Source: CAD feature listing. Evaluate the final solid. Frame: model axes, mm. A direction names the side the tool comes from. Coordinates: 2 decimals unless noted, no trailing zeros. Loops run counter-clockwise (first coordinate to the right, second up) from the corner with the lowest first, then second, coordinate; pieces in that order, holes last. Notation, with made-up numbers: M -36,7.25 L 23,7.25 A20 ccw 23,14.25 Z; hole C -8.75,23.25 d4. An arc over 180 degrees is marked long. One line per question, with ' | ' between items. Start each with the question number.
1. Section query B-B, the plane y = 4.5. Output: boundary loops of the cut face in (x, z).
2. Ray query, probe 1 along X at (y, z) = (3, 6); probe 2 along X at (y, z) = (-5.25, 6); probe 3 along X at (y, z) = (6.5, 6). Return the intervals inside material, ascending.
3. Section query A-A, the plane z = 6. Output: boundary loops of the cut face in (x, y).
4. Access query for faces 5 (the flat face through (9, 0, 1)), 6 (the flat face through (22, 10, 5)). Directions: +Z, -Z, +X, -X, +Y, -Y. A direction counts if a zero-diameter tool reaches every point of the face in a straight line with its end or side. Return the directions, or none.
5. Pin query (flat end, axial travel): P1, Ø4, axis at x = 5, z = 6.5, coming from the +Y side; P2, Ø6.5, axis at x = 12, z = 6, coming from the +Y side; P3, Ø5, axis at x = 17, z = 1.5, coming from the -Y side; P4, Ø1.5, axis at x = 13, y = -2, coming from the -Z side. Return the tip coordinate at first contact, or that it passes through.
6. Section query C-C, the plane x = 4. Output: boundary loops of the cut face in (y, z), and give its area (3 significant figures).
7. Mould query, pull axis Z, two halves, no side actions, for faces 1 (the flat face through (12, 4, 12)), 2 (the flat face through (12, 4, 0)), 3 (the flat face through (14, -10, 8)), 4 (the cylindrical face through (2.8, 5.1, 4.4)). Classes: pulls with the +Z half, pulls with the -Z half, needs draft (parallel to the pull), parting line crosses it, or undercut.
```python
from build123d import *

# Parameters (mm, degrees)
BOSS_EXTRUDE1_DEPTH = 12
SKETCH2_R           = 2
CUT_EXTRUDE1_DEPTH  = 29.635642127
SKETCH3_R           = 4.5
SKETCH3_R_2         = 2.5
BOSS_EXTRUDE2_DEPTH = 10
FILLET1_R           = 1
FILLET2_R           = 0.5


with BuildPart() as part:
    # Sketch1 → Boss-Extrude1 (new body)
    with BuildSketch(Plane.XY):
        with BuildLine():
            Line((17, 10), (24, 10))
            Line((24, 10), (24, 0))
            Line((24, 0), (0, 0))
            Line((0, 0), (0, 10))
            Line((0, 10), (7, 10))
            ThreePointArc((7, 10), (12, 5), (17, 10))
        make_face()
    extrude(amount=BOSS_EXTRUDE1_DEPTH)

    # Sketch2 → Cut-Extrude1 (cut, through all)
    with BuildSketch(Plane(origin=(0, 10, 0), x_dir=(1, 0, 0), z_dir=(0, 1, 0))):
        with Locations(Location((4, -6, 0), (0, 0, 270))):
            Circle(SKETCH2_R)
        with Locations(Location((20, -6, 0), (0, 0, 270))):
            Circle(SKETCH2_R)
    extrude(amount=-CUT_EXTRUDE1_DEPTH, mode=Mode.SUBTRACT)

    # Sketch3 → Boss-Extrude2 (add)
    with BuildSketch(Plane.XZ):
        with Locations(Location((12, 6, 0), (0, 0, 90))):
            Circle(SKETCH3_R)
        with Locations(Location((12, 6, 0), (0, 0, 270))):
            Circle(SKETCH3_R_2, mode=Mode.SUBTRACT)
    extrude(amount=BOSS_EXTRUDE2_DEPTH)

    # Fillet1
    fillet1_edges = [part.edges().sort_by_distance(p)[0] for p in [
        (12, 0, 1.5),
        (12, -10, 1.5),
    ]]
    fillet(fillet1_edges, radius=FILLET1_R)

    # Fillet2
    fillet2_edges = [part.edges().sort_by_distance(p)[0] for p in [
        (24, 0, 6),
        (24, 5, 12),
        (0, 5, 12),
        (24, 5, 0),
        (12, 0, 0),
        (0, 5, 0),
        (12, 0, 12),
    ]]
    fillet(fillet2_edges, radius=FILLET2_R - 0.0001)  # a hair under: the kernel refuses the full size


solid = part.part
```
Taken from the geometry:
1) outline: M 0,0.5 A0.5 ccw 0.5,0 L 23.5,0 A0.5 ccw 24,0.5 L 24,11.5 A0.5 ccw 23.5,12 L 0.5,12 A0.5 ccw 0,11.5 Z; hole C 4,6 d4; hole C 20,6 d4
2) probe 1: 0 to 2, 6 to 18, 22 to 24 | probe 2: 7.5 to 9.5, 14.5 to 16.5 | probe 3: 0 to 2, 6 to 8.43, 15.57 to 18, 22 to 24
3) outline: M 0,0 L 2,0 L 2,10 L 0,10 Z; M 6,0 L 6.5,0 A1 cw 7.5,-1 L 7.5,-9 A1 ccw 8.5,-10 L 9.5,-10 L 9.5,0 L 14.5,0 L 14.5,-10 L 15.5,-10 A1 ccw 16.5,-9 L 16.5,-1 A1 cw 17.5,0 L 18,0 L 18,10 L 17,10 A5 cw 7,10 L 6,10 Z; M 22,0 L 23.5,0 A0.5 ccw 24,0.5 L 24,10 L 22,10 Z
4) face 5: -Y | face 6: +Z, -Z, +X, -X, +Y
5) P1: y = 10 | P2: y = 6.2 | P3: y = -9.69 | P4: z = 1.51
6) outline: M 0,0.5 A0.5 ccw 0.5,0 L 10,0 L 10,4 L 0,4 Z; M 0,8 L 10,8 L 10,12 L 0.5,12 A0.5 ccw 0,11.5 Z | area: 79.9 mm^2
7) face 1: pulls with the +Z half | face 2: pulls with the -Z half | face 3: needs draft | face 4: undercut
